Check sheet for the modelled part. Datum: model origin and axes. Units: mm. Coordinates: 2 decimals unless noted, no trailing zeros. Write each loop counter-clockwise with the first axis right and the second up, starting at its lowest first coordinate (ties: lowest second). Pieces come first, ordered by that corner, then holes. Notation, with made-up numbers: (49.25, 59.25) -> (88.25, 59.25) arc R17 ccw to (88.25, 88.25) -> close; hole circle Ø8 at (-33, 80). An arc over 180 degrees is marked (long way). Put each result on its own line as item: value.
```python
from build123d import *

# Parameters (mm, degrees)
CHAMFER1_SIZE = 0.075


with BuildPart() as part:
    # Sketch1 → Revolve1 (revolve)
    with BuildSketch(Plane.XY):
        with BuildLine():
            Line((-30, 0), (30, 0))
            Line((30, 0), (30, 1))
            Line((30, 1), (21, 1))
            ThreePointArc((21, 1), (19.881966011, 1.126602828), (18.820550528, 1.5))
            ThreePointArc((18.820550528, 1.5), (17.759135045, 1.873397172), (16.641101056, 2))
            Line((16.641101056, 2), (-16.641101056, 2))
            ThreePointArc((-16.641101056, 2), (-17.759135045, 1.873397172), (-18.820550528, 1.5))
            ThreePointArc((-18.820550528, 1.5), (-19.881966011, 1.126602828), (-21, 1))
            Line((-21, 1), (-30, 1))
            Line((-30, 1), (-30, 0))
        make_face()
    revolve(axis=Axis((-30, 0, 0), (1, 0, 0)))

    # Chamfer1
    chamfer1_edges = [part.edges().sort_by_distance(p)[0] for p in [
        (-30, -1, 0),
        (30, -1, 0),
    ]]
    chamfer(chamfer1_edges, length=CHAMFER1_SIZE)


solid = part.part
```
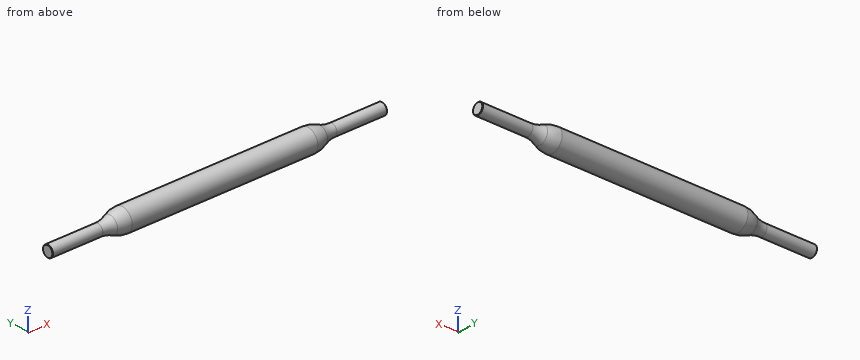
Q1. Cross-section at B-B (x = 4). Record the cut outline in (y, z), plus the area to 3 significant figures.
Recorded:
outline: circle Ø4 at (0, 0)
area: 12.6 mm2
Q2. Material ranges on line 1 along Z through (x, y) = (22.5, 0.1); line 2 along Y through (x, z) = (-25, -0.9); line 3 along Z through (x, y) = (-14.5, 0.1), recorded low to high.
Recorded:
line 1: z = -0.99 to 0.99
line 2: y = -0.44 to 0.44
line 3: z = -2 to 2
Q3. Depth check by flat-ended pin: P1, Ø2, axis at y = 0.5, z = 1, coming from the -X side. Enter the tip coordinate at first touch or a pass-through.
Recorded:
P1: stops at x = -30
Q4. Cross-section at A-A (x = -26). Record the cut outline in (y, z).
Recorded:
outline: circle Ø2 at (0, 0)
